from build123d import *

# Parameters (mm, degrees)
F1_DEPTH = 5.08
F2_R     = 3.175
F3_DEPTH = 25.4
F4_W     = 5.08
F4_H     = 25.4
F5_DEPTH = 5.08


with BuildPart() as f1:
    # F0 (on Right) → F1 (new body)
    with BuildSketch(Plane.YZ):
        Polygon((12.7, 5.08), (12.7, 0), (38.1, 0), (38.1, 5.08), (50.8, 5.08), (50.8, 45.72), (38.1, 45.72), (38.1, 50.8), (12.7, 50.8), (12.7, 45.72), (0, 45.72), (0, 5.08), align=None)
    extrude(amount=F1_DEPTH)

    # F2 (on face) → F3 (cut)
    with BuildSketch(Plane.YZ.offset(5.08)):
        with Locations((25.4, 35.56)):
            Circle(F2_R)
    extrude(amount=-F3_DEPTH, mode=Mode.SUBTRACT)

    # F4 (on face) → F5 (join)
    with BuildSketch(Plane.YZ.offset(5.08)):
        with Locations((-2.54, 26.67)):
            Rectangle(F4_W, F4_H)
        with Locations((53.34, 26.67)):
            Rectangle(F4_W, F4_H)
    extrude(amount=-F5_DEPTH)


solid = f1.part
Read the model definition and answer for the solid it produces. Units are mm, in the model's axes. A direction names the side the tool comes from. Give positions to 0.01 mm unless a question says otherwise; leave off trailing zeros. Write each loop counter-clockwise with the first axis right and the second up, starting at its lowest first coordinate (ties: lowest second). Pieces come first, ordered by that corner, then holes. Notation, with made-up numbers: (43, -39) - (74, -39) arc R25 cw to (74, -4) - close; hole circle Ø2 at (9, 11). An arc over 180 degrees is marked (long way). Use CSV: the item, a comma, the result in double quotes. Start each with the question number.
(1) Consider line 1 along Z through (x, y) = (3, 25.4) (3 decimals); line 2 along Z through (x, y) = (3.5, 10); line 3 along Y through (x, z) = (4.25, 6). Determine where each line is inside the solid, lowest interval first.
(2) For faces 1 (the flat face through (3, 38.1, 3)), 2 (the flat face through (3, 6, 45.72)), 3 (the flat face through (3, 53, 39.37)), determine the directions among +Z, -Z, +X, -X, +Y, -Y from which every point of the face is accessible in a straight line to the end or side of a thin tool.
(3) Find section B-B (x = 1.5). Give the vertices of the cut face in (y, z) (3 decimals), plus the area to 3 significant figures.
(4) Find section A-A (z = 35.56). Give the vertices of the cut face in (x, y) (3 decimals), plus the area to 3 significant figures.
(5) Given P1, Ø1.5, axis at x = 2.5, z = 7.5, coming from the -Y side; P2, Ø1.5, axis at x = 2, y = 41.5, coming from the -Z side; P3, Ø2.5, axis at x = 2, z = 9.5, coming from the +Y side; P4, Ø4, axis at y = 25.4, z = 35.56, coming from the -X side, each flat-ended and moving along its own axis, determine where each tip first touches the part or whether it passes through.
(6) Find section D-D (z = 11). Give the vertices of the cut face in (x, y).
(7) Find section C-C (y = 25.4). Give the vertices of the cut face in (x, z) (3 decimals), plus the area to 3 significant figures.
(8) Determine the mould class of faces 4 (the flat face through (3, 55.88, 26)), 5 (the cylindrical face through (2.576, 26.865, 32.743)), 6 (the flat face through (3, 26, 50.8)) for opening direction Z: +Z half, -Z half, draft (parallel to the pull), parting line (faces both ways), or undercut.
Findings below:
1,line 1,"0 to 32.385, 38.735 to 50.8"
1,line 2,"5.08 to 45.72"
1,line 3,"0 to 50.8"
2,face 1,"-Z, +X, -X, +Y"
2,face 2,"+Z, +X, -X, -Y"
2,face 3,"+Z, +X, -X, +Y"
3,outline,"(-5.08, 13.97) - (0, 13.97) - (0, 5.08) - (12.7, 5.08) - (12.7, 0) - (38.1, 0) - (38.1, 5.08) - (50.8, 5.08) - (50.8, 13.97) - (55.88, 13.97) - (55.88, 39.37) - (50.8, 39.37) - (50.8, 45.72) - (38.1, 45.72) - (38.1, 50.8) - (12.7, 50.8) - (12.7, 45.72) - (0, 45.72) - (0, 39.37) - (-5.08, 39.37) - close; hole circle Ø6.35 at (25.4, 35.56)"
3,area,"2,550 mm2"
4,outline,"(0, -5.08) - (5.08, -5.08) - (5.08, 22.225) - (0, 22.225) - close; (0, 28.575) - (5.08, 28.575) - (5.08, 55.88) - (0, 55.88) - close"
4,area,"277 mm2"
5,P1,"y = 0"
5,P2,"z = 5.08"
5,P3,"y = 50.8"
5,P4,"through"
6,outline,"(0, 0) - (5.08, 0) - (5.08, 50.8) - (0, 50.8) - close"
7,outline,"(0, 0) - (5.08, 0) - (5.08, 32.385) - (0, 32.385) - close; (0, 38.735) - (5.08, 38.735) - (5.08, 50.8) - (0, 50.8) - close"
7,area,"226 mm2"
8,face 4,"draft"
8,face 5,"undercut"
8,face 6,"+Z half"
